Verification items for the finished model (mm, model axes). A direction names the side the tool comes from. Round coordinates to 2 decimals unless told otherwise and drop trailing zeros. Write each loop counter-clockwise with the first axis right and the second up, starting at its lowest first coordinate (ties: lowest second). Pieces come first, ordered by that corner, then holes.
from build123d import *

# Parameters (mm, degrees)
F0_W      = 18
F0_H      = 18
F1_DEPTH  = 7.874
F4_DEPTH  = 25
F5_DEPTH  = 25
F6_T      = -1.6
F7_R      = 2.77
F8_DEPTH  = 7
F10_DEPTH = 3
F11_R     = 0.4


with BuildPart() as f1:
    # F0 (on Top) → F1 (new body)
    with BuildSketch(Plane.XY):
        Rectangle(F0_W, F0_H)
    extrude(amount=F1_DEPTH)

    # F3 (on face) → F4 (cut)
    with BuildSketch(Plane(origin=(-9, 0, 0), x_dir=(0, -1, 0), z_dir=(-1, 0, 0))):
        with BuildLine():
            Line((-6, 7.874), (-9, 7.874))
            Line((-9, 7.874), (-7.232233047, 6.106233047))
            ThreePointArc((-7.232233047, 6.106233047), (-6.6524748606, 7.0154603305), (-6, 7.874))
        make_face()
        with BuildLine():
            Line((-7.232233047, 6.106233047), (-9, 7.874))
            Line((-9, 7.874), (-9, 0))
            ThreePointArc((-9, 0), (-8.491581374, 3.1618143655), (-7.232233047, 6.106233047))
        make_face()
        with BuildLine():
            Line((9, 7.874), (6, 7.874))
            ThreePointArc((6, 7.874), (6.6524748606, 7.0154603305), (7.232233047, 6.106233047))
            Line((7.232233047, 6.106233047), (9, 7.874))
        make_face()
        with BuildLine():
            ThreePointArc((7.232233047, 6.106233047), (8.491581374, 3.1618143655), (9, 0))
            Line((9, 0), (9, 7.874))
            Line((9, 7.874), (7.232233047, 6.106233047))
        make_face()
    extrude(amount=-F4_DEPTH, mode=Mode.SUBTRACT)

    # F2 (on face) → F5 (cut)
    with BuildSketch(Plane.XZ.offset(9)):
        with BuildLine():
            Line((-7.232233047, 6.106233047), (-9, 7.874))
            Line((-9, 7.874), (-9, 0))
            ThreePointArc((-9, 0), (-8.491581374, 3.1618143655), (-7.232233047, 6.106233047))
        make_face()
        with BuildLine():
            Line((-6, 7.874), (-9, 7.874))
            Line((-9, 7.874), (-7.232233047, 6.106233047))
            ThreePointArc((-7.232233047, 6.106233047), (-6.6524748606, 7.0154603305), (-6, 7.874))
        make_face()
        with BuildLine():
            Line((9, 7.874), (6, 7.874))
            ThreePointArc((6, 7.874), (6.6524748606, 7.0154603305), (7.232233047, 6.106233047))
            Line((7.232233047, 6.106233047), (9, 7.874))
        make_face()
        with BuildLine():
            ThreePointArc((7.232233047, 6.106233047), (8.491581374, 3.1618143655), (9, 0))
            Line((9, 0), (9, 7.874))
            Line((9, 7.874), (7.232233047, 6.106233047))
        make_face()
    extrude(amount=-F5_DEPTH, mode=Mode.SUBTRACT)

    # F6
    f6_openings = [f1.faces().sort_by_distance(p)[0] for p in [
        (0, 0, 0),
    ]]
    offset(amount=F6_T, openings=f6_openings)

    # F7 (on face) → F8 (join)
    with BuildSketch(Plane(origin=(0, 0, 0), x_dir=(1, 0, 0), z_dir=(0, 0, -1))):
        Circle(F7_R)
        Polygon((0.7, 2.1), (0.7, 0.7), (2.1, 0.7), (2.1, 0), (2.1, -0.7), (0.7, -0.7), (0.7, -2.1), (0, -2.1), (-0.7, -2.1), (-0.7, -0.7), (-2.1, -0.7), (-2.1, 0), (-2.1, 0.7), (-0.7, 0.7), (-0.7, 2.1), (0, 2.1), align=None, mode=Mode.SUBTRACT)
    extrude(amount=-F8_DEPTH)

    # F9 (on face) → F10 (cut)
    with BuildSketch(Plane(origin=(0, 0, 0), x_dir=(1, 0, 0), z_dir=(0, 0, -1))):
        with BuildLine():
            Line((-2.1, -0.7), (-2.1, 0.7))
            Line((-2.1, 0.7), (-2.680093282, 0.7))
            ThreePointArc((-2.680093282, 0.7), (-2.77, 0), (-2.680093282, -0.7))
            Line((-2.680093282, -0.7), (-2.1, -0.7))
        make_face()
        with BuildLine():
            ThreePointArc((2.77, 0), (2.7474313814, 0.3528750551), (2.680093282, 0.7))
            Line((2.680093282, 0.7), (2.1, 0.7))
            Line((2.1, 0.7), (2.1, -0.7))
            Line((2.1, -0.7), (2.680093282, -0.7))
            ThreePointArc((2.680093282, -0.7), (2.7474313814, -0.3528750551), (2.77, 0))
        make_face()
    extrude(amount=-F10_DEPTH, mode=Mode.SUBTRACT)

    # F11
    f11_edges = [f1.edges().sort_by_distance(p)[0] for p in [
        (6, 0, 7.874),
        (0, -6, 7.874),
        (0, 6, 7.874),
        (-6, 0, 7.874),
        (8.078099, 8.078099, 4.367421),
        (8.078099, -8.078099, 4.367421),
        (-8.078099, -8.078099, 4.367421),
        (-8.078099, 8.078099, 4.367421),
    ]]
    fillet(f11_edges, radius=F11_R)

    # F12 (on Front) → F13 (revolve, cut)
    with BuildSketch(Plane.XZ):
        with BuildLine():
            ThreePointArc((-10, 10), (-5.2316729526, 7.7080140656), (0, 6.9207780963))
            Line((0, 6.9207780963), (0, 10))
            Line((0, 10), (-10, 10))
        make_face()
    revolve(axis=Axis((0, 0, 5), (0, 0, 1)), mode=Mode.SUBTRACT)


solid = f1.part
Q1. Material ranges on line 1 along Y through (x, z) = (1.25, 4.5); line 2 along Y through (x, z) = (-0.25, 5); line 3 along X through (y, z) = (-1.75, 1.25), recorded low to high.
Recorded:
line 1: y = -8.02 to -6.27, -2.47 to -0.7, 0.7 to 2.47, 6.27 to 8.02
line 2: y = -7.81 to -6.02, -2.76 to -2.1, 2.1 to 2.76, 6.02 to 7.81
line 3: x = -8.89 to -7.28, -2.15 to -0.7, 0.7 to 2.15, 7.28 to 8.89
Q2. Sectioned sample at A-A (y = 0). Enter the section's corners in (x, z), plus the area to 3 significant figures.
Recorded:
outline: (-9, 0) - (-7.4, 0) arc R11.52 cw to (-5.22, 6.27) - (-2.77, 6.27) - (-2.77, 3) - (-2.1, 3) - (-2.1, 6.27) - (2.1, 6.27) - (2.1, 3) - (2.77, 3) - (2.77, 6.27) - (5.22, 6.27) arc R11.52 cw to (7.4, 0) - (9, 0) arc R13.12 ccw to (6.12, 7.72) arc R0.4 ccw to (5.81, 7.87) - (5.74, 7.87) arc R17.78 cw to (-5.74, 7.87) - (-5.81, 7.87) arc R0.4 ccw to (-6.12, 7.72) arc R13.12 ccw to start
area: 39.5 mm2
Q3. Tool access check on faces 1 (the flat face through (0.7, -1, 3)), 2 (the flat face through (-8, 0, 0)). Record the directions out of +Z, -Z, +X, -X, +Y, -Y that give a thin tool (end or side, any length) a straight path to the whole face; none if there is none.
Recorded:
face 1: -Z
face 2: -Z, +X, -X, +Y, -Y
Q4. Sectioned sample at C-C (z = 2.25). Give the number of separate pieces and of enclosed holes in the cut face, plus the area to 3 significant figures.
Recorded:
separate pieces: 3
enclosed holes: 1
area: 116 mm2
Q5. Sectioned sample at D-D (x = 5). Enter the section's corners in (y, z).
Recorded:
outline: (-9, 0) - (-7.4, 0) arc R11.52 cw to (-5.22, 6.27) - (5.22, 6.27) arc R11.52 cw to (7.4, 0) - (9, 0) arc R13.12 ccw to (6.12, 7.72) arc R0.4 ccw to (5.81, 7.87) - (2.83, 7.87) arc R17.06 cw to (-2.83, 7.87) - (-5.81, 7.87) arc R0.4 ccw to (-6.12, 7.72) arc R13.12 ccw to start
Q6. Release check for a two-part mould opening along Y. For faces 3 (the flat face through (0, 2.4, 0)), 4 (the flat face through (2.1, 0, 5)) record: released by +Y, released by -Y, zero draft, split by the parting line, or undercut.
Recorded:
face 3: zero draft
face 4: undercut
Q7. Sectioned sample at B-B (x = 0). Enter the section's corners in (y, z), plus the area to 3 significant figures.
Recorded:
outline: (-9, 0) - (-7.4, 0) arc R11.52 cw to (-5.22, 6.27) - (-2.77, 6.27) - (-2.77, 0) - (-2.1, 0) - (-2.1, 6.27) - (2.1, 6.27) - (2.1, 0) - (2.77, 0) - (2.77, 6.27) - (5.22, 6.27) arc R11.52 cw to (7.4, 0) - (9, 0) arc R13.12 ccw to (6.12, 7.72) arc R0.4 ccw to (5.81, 7.87) - (5.74, 7.87) arc R17.78 cw to (-5.74, 7.87) - (-5.81, 7.87) arc R0.4 ccw to (-6.12, 7.72) arc R13.12 ccw to start
area: 43.5 mm2
Q8. Depth check by flat-ended pin: P1, Ø8, axis at x = 7, y = 7, coming from the -Z side; P2, Ø1, axis at x = -2, z = 4, coming from the -Y side; P3, Ø1, axis at x = -1.5, z = 4.5, coming from the +Y side; P4, Ø1.5, axis at y = 0, z = 4, coming from the -X side. Enter the tip coordinate at first touch or a pass-through.
Recorded:
P1: stops at z = 0
P2: stops at y = -8.39
P3: stops at y = 8.22
P4: stops at x = -8.47
